from build123d import *

# Parameters (mm, degrees)
F0_W     = 100
F0_H     = 100
F1_DEPTH = 25
F2_W     = 20
F2_H     = 20
F3_DEPTH = 100
F4_W     = 100
F4_H     = 7.817208
F5_DEPTH = 150


with BuildPart() as f1:
    # F0 (on Top) → F1 (new body)
    with BuildSketch(Plane.XY):
        with Locations((0.650306, -2.683234)):
            Rectangle(F0_W, F0_H)
    extrude(amount=F1_DEPTH)

    # F2 (on Top) → F3 (join)
    with BuildSketch(Plane.XY):
        with Locations((33.802878, 34.537725)):
            Rectangle(F2_W, F2_H)
        with Locations((33.802878, -37.14768)):
            Rectangle(F2_W, F2_H)
        with Locations((-35.945089, 34.537725)):
            Rectangle(F2_W, F2_H)
        with Locations((-35.945089, -39.085125)):
            Rectangle(F2_W, F2_H)
    extrude(amount=-F3_DEPTH)

    # F4 (on Top) → F5 (join)
    with BuildSketch(Plane.XY):
        with Locations((0.545476, 43.83298)):
            Rectangle(F4_W, F4_H)
    extrude(amount=F5_DEPTH)


solid = f1.part
Work out the finished part from the listing and answer in its coordinate system (mm). A direction names the side the tool comes from. Round coordinates to 2 decimals unless told otherwise and drop trailing zeros. Loops run counter-clockwise (first coordinate to the right, second up) from the corner with the lowest first, then second, coordinate; pieces in that order, holes last. Notation, with made-up numbers: M -5,53.5 L 39,53.5 A23 ccw 39,69.5 Z; hole C 4.5,87.5 d7. An arc over 180 degrees is marked long. One line per question, with ' | ' between items. Start each with the question number.
(1) A cutting plane is placed at C-C on y = 34. Write down the section's boundary in (x, z).
(2) A cutting plane is placed at B-B on x = 40. Write down the section's boundary in (y, z).
(3) A cutting plane is placed at A-A on z = -50.5. Write down the section's boundary in (x, y), plus the area to 3 significant figures.
(4) Flat-ended cylindrical pins translate along their axes: pin 1 Ø10 at (x, z) = (31, -42) entering from -Y; pin 2 Ø22 at (y, z) = (-35, -52.5) entering from -X; pin 3 Ø4 at (x, y) = (23, -6.5) entering from +Z. Find the tip coordinate at first contact, or state that the pin passes through.
(5) Find the intervals of material crossed by line 1 (Z direction, x = 17.5, y = -45.5); line 2 (Y direction, x = 33.5, z = 74); line 3 (Z direction, x = -30.5, y = 39), in increasing order.
(6) For a pull along X with two mould halves and no side action, classify faces 1 (the face through (-25.945, 34, -49)), 2 (the face through (-36, -29.085, -49)), 3 (the face through (-25.945, -39, -49)), 4 (the face through (-45.945, 34, -49)) as released by +X, released by -X, zero draft, split by the parting line, or undercut.
(7) A cutting plane is placed at D-D on z = 127.5. Write down the section's boundary in (x, y).
(8) A tool of negligible diameter and unlimited length cuts with its end or side. For faces 5 (the face through (23.803, 34, -49)), 6 (the face through (-36, -49.085, -49)), 7 (the face through (43.803, -37, -49)), 8 (the face through (-36, 44.538, -49)), 9 (the face through (34, -27.148, -49)), from which of +Z, -Z, +X, -X, +Y, -Y can it reach the whole face along a straight path? Write none if from no direction.
Geometry check:
1) outline: M -49.35,0 L -45.95,0 L -45.95,-100 L -25.95,-100 L -25.95,0 L 23.8,0 L 23.8,-100 L 43.8,-100 L 43.8,0 L 50.65,0 L 50.65,25 L -49.35,25 Z
2) outline: M -52.68,0 L -47.15,0 L -47.15,-100 L -27.15,-100 L -27.15,0 L 24.54,0 L 24.54,-100 L 44.54,-100 L 44.54,0 L 47.74,0 L 47.74,150 L 39.92,150 L 39.92,25 L -52.68,25 Z
3) outline: M -45.95,-49.09 L -25.95,-49.09 L -25.95,-29.09 L -45.95,-29.09 Z; M -45.95,24.54 L -25.95,24.54 L -25.95,44.54 L -45.95,44.54 Z; M 23.8,-47.15 L 43.8,-47.15 L 43.8,-27.15 L 23.8,-27.15 Z; M 23.8,24.54 L 43.8,24.54 L 43.8,44.54 L 23.8,44.54 Z | area: 1,600 mm²
4) pin 1: stops at y = -47.15 | pin 2: stops at x = -45.95 | pin 3: stops at z = 25
5) line 1: z = 0 to 25 | line 2: y = 39.92 to 47.74 | line 3: z = -100 to 25
6) face 1: undercut | face 2: zero draft | face 3: undercut | face 4: released by -X
7) outline: M -49.45,39.92 L 50.55,39.92 L 50.55,47.74 L -49.45,47.74 Z
8) face 5: -Z, +Y, -Y | face 6: -Z, +X, -X, -Y | face 7: -Z, +X, +Y, -Y | face 8: -Z, +X, -X, +Y | face 9: -Z, +X, -X
